```python
from build123d import *


with BuildPart() as f2:
    # F2: sweep along a path in F0
    with BuildLine(Plane.XY) as f2_path:
        Line((-200, -82.8427124746), (-200, 82.8427124746))
        Line((-200, 82.8427124746), (-82.8427124746, 200))
        Line((-82.8427124746, 200), (82.8427124746, 200))
        Line((82.8427124746, 200), (200, 82.8427124746))
        Line((200, 82.8427124746), (200, -82.8427124746))
        Line((200, -82.8427124746), (82.8427124746, -200))
        Line((82.8427124746, -200), (-82.8427124746, -200))
        Line((-82.8427124746, -200), (-200, -82.8427124746))
    # F1 (on Front) → F2 (sweep)
    with BuildSketch(Plane.XZ):
        Polygon((-150, 0), (-200, 0), (-200, -50), (-195, -50), (-195, -5), (-150, -5), align=None)
    sweep(path=f2_path.line, transition=Transition.RIGHT)


solid = f2.part
```
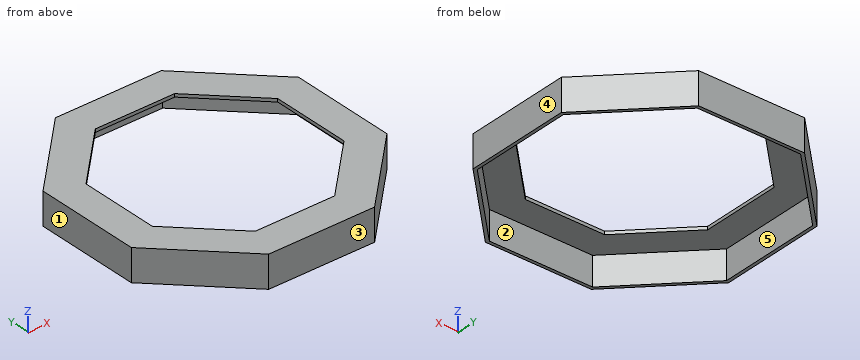
Build history of the part. All positions in model axes, mm. Face numbers are marked on the shaded views. A direction names the side the tool comes from. Give positions to 0.01 mm unless a question says otherwise; leave off trailing zeros. Loops run counter-clockwise (first coordinate to the right, second up) from the corner with the lowest first, then second, coordinate; pieces in that order, holes last. Notation, with made-up numbers: (-10, 89.5) -> (22, 89.5) arc R22 ccw to (22, 111.5) -> close; hole circle Ø5 at (35, 56.5). An arc over 180 degrees is marked (long way). One line per question, with ' | ' between items.
Q1. Tool access for the marked faces 4 and 5: list every direction of +Z, -Z, +X, -X, +Y, -Y with a clear straight run to the whole face (end or side of a thin tool).
Filled sheet:
face 4: +Z, -Z, +X, +Y, -Y | face 5: -Z
Q2. Drop flat-ended pins along their axis: pin 1 (3 mm diameter, centred on x = -124, y = 120.5, fed in from -Z); pin 2 (12 mm diameter, centred on x = 107.5, z = -8, fed in from -Y); pin 3 (12 mm diameter, centred on y = 110.5, z = -23.5, fed in from +X). Give the stop position or say it passes through.
Filled sheet:
pin 1: stops at z = -5 | pin 2: stops at y = -181.34 | pin 3: stops at x = 178.34
Q3. Cut at A-A, the plane y = -36. Write the cut outline in (x, z).
Filled sheet:
outline: (-200, -50) -> (-195, -50) -> (-195, -5) -> (-150, -5) -> (-150, 0) -> (-200, 0) -> close; (150, -5) -> (195, -5) -> (195, -50) -> (200, -50) -> (200, 0) -> (150, 0) -> close
Q4. Cut at C-C, the plane z = -26.5. Write the cut outline in (x, y), plus the area to 3 significant figures.
Filled sheet:
outline: (-200, -82.84) -> (-82.84, -200) -> (82.84, -200) -> (200, -82.84) -> (200, 82.84) -> (82.84, 200) -> (-82.84, 200) -> (-200, 82.84) -> close; hole (-195, -80.77) -> (-80.77, -195) -> (80.77, -195) -> (195, -80.77) -> (195, 80.77) -> (80.77, 195) -> (-80.77, 195) -> (-195, 80.77) -> close | area: 6,540 mm²
Q5. Drill centre lines: line 1 along X through (y, z) = (-34, -46.5); line 2 along X through (y, z) = (-30, -3). Where is each one in solid material? Low to high. Write a range as [from, to].
Filled sheet:
line 1: x = [-200, -195], [195, 200] | line 2: x = [-200, -150], [150, 200]
Q6. Cut at D-D, the plane y = 164. Write the cut outline in (x, z), plus the area to 3 significant figures.
Filled sheet:
outline: (-118.84, -50) -> (-111.77, -50) -> (-111.77, -5) -> (111.77, -5) -> (111.77, -50) -> (118.84, -50) -> (118.84, 0) -> (-118.84, 0) -> close | area: 1,820 mm²
Q7. Pull direction X, two halves, no side cores. Call the marked faces 1, 2 and 3: pulls with the +X half, pulls with the -X half, needs draft (parallel to the pull), parting line crosses it, or undercut.
Filled sheet:
face 1: pulls with the -X half | face 2: undercut | face 3: needs draft
